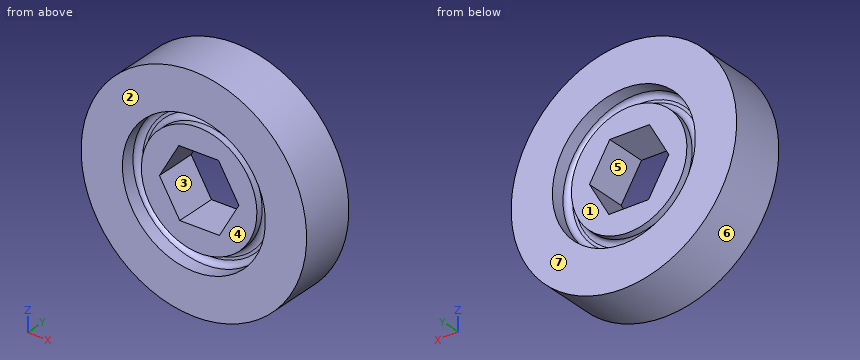
```python
from build123d import *

# Parameters (mm, degrees)
SKETCH1_R               = 20.5
BOSS_EXTRUDE1_DEPTH     = 10
SKETCH2_R               = 13
CUT_EXTRUDE1_DEPTH      = 3.5
CUT_EXTRUDE2_START      = -3.5
SKETCH3_R               = 13
CUT_EXTRUDE2_DEPTH      = 3.5
SKETCH5_R               = 10.5
BOSS_EXTRUDE2_DEPTH     = 2.25
BOSS_EXTRUDE3_START     = 2.25
SKETCH6_R               = 10.5
BOSS_EXTRUDE3_DEPTH     = 2.25
CUT_EXTRUDE3_DEPTH      = 30.711109033
CUT_EXTRUDE3_DEPTH_BACK = 30.711109033
FILLET1_R               = 1
FILLET2_R               = 1


with BuildPart() as part:
    # Sketch1 → Boss-Extrude1 (new body)
    with BuildSketch(Plane(origin=(0, 0, 0), x_dir=(1, 0, 0), z_dir=(0, 1, 0))):
        with Locations(Location((0, 0, 0), (0, 0, 270))):
            Circle(SKETCH1_R)
    extrude(amount=BOSS_EXTRUDE1_DEPTH)

    # Sketch2 → Cut-Extrude1 (cut)
    with BuildSketch(Plane(origin=(0, 10, 0), x_dir=(1, 0, 0), z_dir=(0, 1, 0))):
        with Locations(Location((0, 0, 0), (0, 0, 270))):
            Circle(SKETCH2_R)
    extrude(amount=-CUT_EXTRUDE1_DEPTH, mode=Mode.SUBTRACT)

    # Sketch3 → Cut-Extrude2 (cut)
    with BuildSketch(Plane.XZ.offset(CUT_EXTRUDE2_START)):
        with Locations(Location((0, 0, 0), (0, 0, 90))):
            Circle(SKETCH3_R)
    extrude(amount=CUT_EXTRUDE2_DEPTH, mode=Mode.SUBTRACT)

    # Sketch5 → Boss-Extrude2 (add)
    with BuildSketch(Plane(origin=(0, 6.5, 0), x_dir=(1, 0, 0), z_dir=(0, 1, 0))):
        with Locations(Location((0, 0, 0), (0, 0, 270))):
            Circle(SKETCH5_R)
    extrude(amount=BOSS_EXTRUDE2_DEPTH)

    # Sketch6 → Boss-Extrude3 (add)
    with BuildSketch(Plane.XZ.offset(-3.5).offset(BOSS_EXTRUDE3_START)):
        with Locations(Location((0, 0, 0), (0, 0, 90))):
            Circle(SKETCH6_R)
    extrude(amount=-BOSS_EXTRUDE3_DEPTH)

    # Sketch4 → Cut-Extrude3 (cut, two sides: drawn at the far end of the back side and taken through both)
    with BuildSketch(Plane(origin=(0, 6.5, 0), x_dir=(1, 0, 0), z_dir=(0, 1, 0)).offset(-CUT_EXTRUDE3_DEPTH_BACK)):
        Polygon((3.689639098, 6.202410552), (-3.526625554, 6.296526466), (-7.216264652, 0.094115913), (-3.689639098, -6.202410552), (3.526625554, -6.296526466), (7.216264652, -0.094115913), align=None)
    extrude(amount=CUT_EXTRUDE3_DEPTH + CUT_EXTRUDE3_DEPTH_BACK, mode=Mode.SUBTRACT)

    # Fillet1
    fillet1_edges = [part.edges().sort_by_distance(p)[0] for p in [
        (0, 3.5, -13),
        (0, 6.5, -13),
    ]]
    fillet(fillet1_edges, radius=FILLET1_R)

    # Fillet2
    fillet2_edges = [part.edges().sort_by_distance(p)[0] for p in [
        (0, 6.5, -10.5),
        (0, 3.5, -10.5),
    ]]
    fillet(fillet2_edges, radius=FILLET2_R)


solid = part.part
```
Could you check a few things on this model? Use its own coordinates, in mm. Face numbers are marked on the shaded views. A direction names the side the tool comes from. Round coordinates to 2 decimals unless told otherwise and drop trailing zeros. Loops run counter-clockwise (first coordinate to the right, second up) from the corner with the lowest first, then second, coordinate; pieces in that order, holes last.
Q1. For P1, Ø3, axis at y = 2.5, z = 5, coming from the -X side; P2, Ø6, axis at x = -6.5, z = -7.5, coming from the -Y side; P3, Ø4, axis at y = 2, z = 6, coming from the -X side; P4, Ø3, axis at x = 2.5, z = -2.5, coming from the -Y side, each with a flat end and sliding along its axis, tell me the tip position at first contact or that it passes through.
Q2. On a 3-axis mill with a long thin cutter (end or side, diameter ignored), from which of +Z, -Z, +X, -X, +Y, -Y can I reach the whole of each face in a straight line? I mean the marked faces 1, 2, 3 and 4. Say none if no direction works.
Q3. Thinking about a two-plate mould opening in X: for the marked faces 5, 6 and 7, which applies, pulls with the +X half, pulls with the -X half, needs draft (parallel to the pull), parting line crosses it, or undercut?
Q4. Please list where these lines run through material, in increasing order: L1, parallel to X at y = 9.05, z = 0; L2, parallel to X at y = 3, z = -9; L3, parallel to Z at x = -10, y = 1.
Q5. I want a section at D-D (z = -16). Write out the boundary of the cut face in (x, y).
Q6. I want a section at A-A (y = 5.5). Write out the boundary of the cut face in (x, z), and give its area (3 significant figures).
Q7. I want a section at C-C (x = -17). Write out the boundary of the cut face in (y, z).
Answer below:
1. P1: stops at x = -20.2
1. P2: stops at y = 1.25
1. P3: stops at x = -20.11
1. P4: passes through
2. face 1: +Y
2. face 2: +Z, -Z, +X, -X, -Y
2. face 3: +Y, -Y
2. face 4: -Y
3. face 5: undercut
3. face 6: parting line crosses it
3. face 7: needs draft
4. L1: x = -20.5 to -13, 13 to 20.5
4. L2: x = -18.42 to -9.19, -5.66 to 5.66, 9.19 to 18.42
4. L3: z = -17.9 to -8.31, 8.31 to 17.9
5. outline: (-12.82, 0) - (12.82, 0) - (12.82, 10) - (-12.82, 10) - close
6. outline: circle Ø41 at (0, 0); hole (-7.22, -0.09) - (-3.53, -6.3) - (3.69, -6.2) - (7.22, 0.09) - (3.53, 6.3) - (-3.69, 6.2) - close
6. area: 1,180 mm2
7. outline: (0, -11.46) - (10, -11.46) - (10, 11.46) - (0, 11.46) - close
